Check sheet for the modelled part. Datum: model origin and axes. Units: mm. A direction names the side the tool comes from. Give positions to 0.01 mm unless a question says otherwise; leave off trailing zeros. Order: outer loops, then holes, each group sorted by start corner. A loop starts at its lowest first (then second) coordinate and runs counter-clockwise, first axis right, second up. Notation, with made-up numbers: M 66,63.25 L 89,63.25 A13 cw 89,76.25 Z; hole C 10.5,80.5 d3. An arc over 180 degrees is marked long. One line per question, with ' | ' between items. Start each with the question number.
```python
from build123d import *

# Parameters (mm, degrees)
IZIM1_R                     = 43.965787967
Y_KSEKLIK_EKSTR_ZYON1_DEPTH = 3
IZIM1_3_R                   = 42.5
IZIM1_3_R_2                 = 32.5
EKSTR_ZYON_NCE1_DEPTH       = 5
RADYUS1_R                   = 10
KES_EKSTR_ZYON1_DEPTH       = 3.0000001
KES_EKSTR_ZYON1_DEPTH_BACK  = 4.0000001
KES_EKSTR_ZYON2_DEPTH       = 2
KES_EKSTR_ZYON3_DEPTH       = 3.0000001
IZIM6_R                     = 20.5
KES_EKSTR_ZYON4_DEPTH       = 4.0000001
Y_KSEKLIK_EKSTR_ZYON4_DEPTH = 3


with BuildPart() as part:
    # Çizim1 → Yükseklik-Ekstrüzyon1 (new body)
    with BuildSketch(Plane(origin=(0, 0, 0), x_dir=(1, 0, 0), z_dir=(0, 1, 0))):
        Circle(IZIM1_R)
    extrude(amount=Y_KSEKLIK_EKSTR_ZYON1_DEPTH)

    # Çizim1<3> → Ekstrüzyon-İnce1 (add)
    with BuildSketch(Plane(origin=(0, 0, 0), x_dir=(1, 0, 0), z_dir=(0, 1, 0))):
        with Locations((76.459347515, -0.992424829)):
            Circle(IZIM1_3_R)
        with Locations((76.459347515, -0.992424829)):
            Circle(IZIM1_3_R_2, mode=Mode.SUBTRACT)
        with Locations((-0.992424829, -76.459347515)):
            Circle(IZIM1_3_R)
        with Locations((-0.992424829, -76.459347515)):
            Circle(IZIM1_3_R_2, mode=Mode.SUBTRACT)
        with Locations((-76.459347515, 0.992424829)):
            Circle(IZIM1_3_R)
        with Locations((-76.459347515, 0.992424829)):
            Circle(IZIM1_3_R_2, mode=Mode.SUBTRACT)
        with Locations((0.992424829, 76.459347515)):
            Circle(IZIM1_3_R)
        with Locations((0.992424829, 76.459347515)):
            Circle(IZIM1_3_R_2, mode=Mode.SUBTRACT)
    extrude(amount=EKSTR_ZYON_NCE1_DEPTH)

    # Radyus1
    radyus1_edges = [part.edges().sort_by_distance(p)[0] for p in [
        (-20.683952175, 1.5, 38.796451307),
        (19.670015447, 1.5, 39.320236569),
        (38.796451307, 1.5, 20.683952175),
        (39.320236569, 1.5, -19.670015447),
        (20.683952175, 1.5, -38.796451307),
        (-19.670015447, 1.5, -39.320236569),
        (-38.796451307, 1.5, -20.683952175),
        (-39.320236569, 1.5, 19.670015447),
    ]]
    fillet(radyus1_edges, radius=RADYUS1_R)

    # Çizim3 → Kes-Ekstrüzyon1 (cut, two sides)
    with BuildSketch(Plane(origin=(0, 3, 0), x_dir=(1, 0, 0), z_dir=(0, 1, 0))) as kes_ekstr_zyon1_sk:
        with BuildLine():
            Line((69.327141955, 36.841179861), (69.327141955, 33.783740052))
            ThreePointArc((69.327141955, 33.783740052), (111.959347515, -0.992424829), (69.327141955, -35.76858971))
            Line((69.327141955, -35.76858971), (69.327141955, -38.826029519))
            ThreePointArc((69.327141955, -38.826029519), (114.959347515, -0.992424829), (69.327141955, 36.841179861))
        make_face()
    extrude(amount=KES_EKSTR_ZYON1_DEPTH, mode=Mode.SUBTRACT)
    extrude(kes_ekstr_zyon1_sk.sketch, amount=-KES_EKSTR_ZYON1_DEPTH_BACK, mode=Mode.SUBTRACT)

    # Çizim4 → Kes-Ekstrüzyon2 (cut)
    with BuildSketch(Plane(origin=(0, 5, 0), x_dir=(1, 0, 0), z_dir=(0, 1, 0))):
        Polygon((48.909390592, -25.92206781), (55.608378692, -25.92206781), (55.608378692, 23.937218152), (48.909390592, 23.937218152), (48.909390592, 40.294217079), (36.28293528, 40.294217079), (36.28293528, 23.937218152), (27.96095337, 23.937218152), (27.96095337, -25.92206781), (36.28293528, -25.92206781), (36.28293528, -39.195058406), (48.909390592, -39.195058406), align=None)
    extrude(amount=-KES_EKSTR_ZYON2_DEPTH, mode=Mode.SUBTRACT)

    # Çizim3<4> → Kes-Ekstrüzyon3 (cut, through all)
    with BuildSketch(Plane(origin=(0, 3, 0), x_dir=(1, 0, 0), z_dir=(0, 1, 0))):
        with BuildLine():
            ThreePointArc((47.215527353, -26.033370944), (57.179387966, -34.317087765), (69.327141955, -38.826029519))
            Line((69.327141955, -38.826029519), (69.327141955, -35.76858971))
            ThreePointArc((69.327141955, -35.76858971), (58.437150617, -31.577558783), (49.494266586, -24.08212839))
            Line((49.494266586, -24.08212839), (47.215527353, -26.033370944))
        make_face()
        with BuildLine():
            Line((69.327141955, 33.783740052), (69.327141955, 36.841179861))
            ThreePointArc((69.327141955, 36.841179861), (57.316539714, 32.411211343), (47.42238732, 24.288100138))
            Line((47.42238732, 24.288100138), (49.685007595, 22.318189102))
            ThreePointArc((49.685007595, 22.318189102), (58.563030261, 29.666535179), (69.327141955, 33.783740052))
        make_face()
    extrude(amount=KES_EKSTR_ZYON3_DEPTH, mode=Mode.SUBTRACT)

    # Çizim6 → Kes-Ekstrüzyon4 (cut, through all)
    with BuildSketch(Plane(origin=(0, 3, 0), x_dir=(1, 0, 0), z_dir=(0, 1, 0))):
        Circle(IZIM6_R)
    extrude(amount=-KES_EKSTR_ZYON4_DEPTH, mode=Mode.SUBTRACT)

    # Çizim3<6> → Yükseklik-Ekstrüzyon4 (add)
    with BuildSketch(Plane(origin=(0, 3, 0), x_dir=(1, 0, 0), z_dir=(0, 1, 0))):
        with BuildLine():
            ThreePointArc((34.591220847, -8.293792461), (39.7514282, -5.784707132), (41.840982512, -0.44083102))
            ThreePointArc((41.840982512, -0.44083102), (39.820297101, 4.827467905), (34.794834124, 7.39317735))
            ThreePointArc((34.794834124, 7.39317735), (33.962927145, -0.44083102), (34.591220847, -8.293792461))
        make_face()
        with BuildLine():
            ThreePointArc((34.591220847, -8.293792461), (33.962927145, -0.44083102), (34.794834124, 7.39317735))
            ThreePointArc((34.794834124, 7.39317735), (26.08553532, -0.338584277), (34.591220847, -8.293792461))
        make_face()
    extrude(amount=Y_KSEKLIK_EKSTR_ZYON4_DEPTH)


solid = part.part
```
Item 1: Section check C-C, the plane z = -55. Record the cut outline in (x, y).
Item 2: Go/stop test with flat-tipped pins: P1, Ø1, axis at x = 84.5, y = 5, coming from the -Z side; P2, Ø1, axis at y = 2.5, z = -28, coming from the +X side; P3, Ø2, axis at x = 53.5, y = 3.5, coming from the -Z side; P4, Ø5, axis at x = 25.5, z = -93.5, coming from the -Y side. Record where each tip stops, or that it passes through.
Item 3: Section check D-D, the plane x = 82.5. Record the cut outline in (y, z), then the cut area to 3 significant figures.
Item 4: Draft check along Z on faces 1 (the face through (118.914, 2.465, 2.947)), 2 (the face through (-27, 0, -1)), 3 (the face through (-10.206, 2.465, 117.949)). Enter one of: released by +Z, released by -Z, zero draft, split by the parting line, or undercut.
Item 5: Set-up check for faces 4 (the face through (34, 6, 0)), 5 (the face through (-86.1, 5, 30.3)), 6 (the face through (-9, 5, -45)), 7 (the face through (-8.038, 2.465, 108.187)), 8 (the face through (-11, 5, 108)): record each of +Z, -Z, +X, -X, +Y, -Y from which the full face is reachable in a straight line by a thin tool's end or side.
Item 6: Scan lines: probe 1 along X at (y, z) = (0.8, 0); probe 2 along Z at (x, y) = (0, 2.1); probe 3 along X at (y, z) = (3.5, -29). Record each from-to range of solid material in increasing order. Write a range as [from, to].
Item 7: Section check B-B, the plane y = 4. State how many separate pieces and enclosed holes the cut face has, then the cut area to 3 significant figures.
Item 8: Section check A-A, the plane x = -89.5. Record the cut outline in (y, z).
Reported:
1) outline: M -35.69,0 L -23.42,0 L -23.42,5 L -35.69,5 Z; M 25.4,0 L 37.68,0 L 37.68,5 L 25.4,5 Z
2) P1: stops at z = -40.83 | P2: stops at x = 107.99 | P3: stops at z = -35.39 | P4: passes through
3) outline: M 0,-41.08 L 5,-41.08 L 5,-37.03 L 0,-37.03 Z; M 0,-33.99 L 5,-33.99 L 5,-30.94 L 0,-30.94 Z; M 0,32.93 L 5,32.93 L 5,35.97 L 0,35.97 Z; M 0,39.02 L 5,39.02 L 5,43.06 L 0,43.06 Z | area: 70.9 mm^2
4) face 1: split by the parting line | face 2: zero draft | face 3: undercut
5) face 4: +Z, -Z, +X, -X, +Y | face 5: +Z, -Z, -X, +Y | face 6: -Z, +X, -X, +Y | face 7: +Y, -Y | face 8: +Z, +X, -X, +Y
6) probe 1: x = [-118.95, -108.94], [-43.97, -20.5], [20.5, 43.97], [108.94, 111.95], [114.95, 118.95] | probe 2: z = [-118.95, -108.94], [-43.97, -20.5], [20.5, 43.97], [108.94, 118.95] | probe 3: x = [-108.43, -92.95], [-59.97, -44.49], [48.91, 52.32], [57.47, 63.94], [88.98, 95.45], [100.6, 106.57]
7) separate pieces: 6 | enclosed holes: 3 | area: 8,490 mm^2
8) outline: M 0,-41.44 L 5,-41.44 L 5,-30.76 L 0,-30.76 Z; M 0,28.78 L 5,28.78 L 5,39.46 L 0,39.46 Z
